Source: CAD feature listing. Evaluate the final solid. Frame: model axes, mm. Face numbers are marked on the shaded views. Round coordinates to 2 decimals unless told otherwise and drop trailing zeros. Order: outer loops, then holes, each group sorted by start corner. A loop starts at its lowest first (then second) coordinate and runs counter-clockwise, first axis right, second up. Notation, with made-up numbers: M -19,9 L 21,9 A27 cw 21,44 Z; hole C -10.75,-2.5 d10. An arc over 180 degrees is marked long. Use one line per item in the form item = value. Start each with the question number.
Q1. Section B-B (y = 0). Return the cut outline in (x, z).
Q2. Pull-direction query (Z, two-part tool) for the marked faces 1, 2 and 3; classes: pulls with the +Z half, pulls with the -Z half, needs draft (parallel to the pull), parting line crosses it, or undercut.
Q3. Contact query for flat-ended pins moving along their axis: pin 1 (3 mm diameter, centred on x = -41.5, y = -52, fed in from -Z); pin 2 (5 mm diameter, centred on y = -3.5, z = 354.5, fed in from +X); pin 3 (12 mm diameter, centred on x = 9.5, z = 331, fed in from -Y). Output: stop coordinate, or through.
Q4. Section A-A (x = 33). Return the cut outline in (y, z).
Q5. Section C-C (y = -29.5). Return the cut outline in (x, z), plus the area to 3 significant figures.
Q6. Material intervals for probe 1 along Z at (x, y) = (-42, 3.5); probe 2 along X at (y, z) = (2, 22); probe 3 along X at (y, z) = (-0.5, 442), sorted ascending.
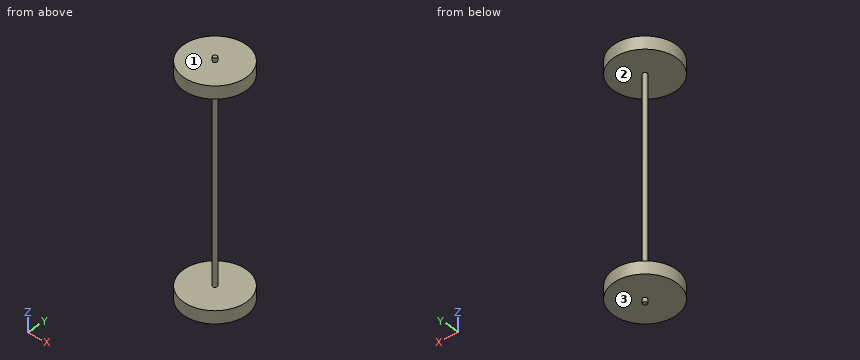
Autodesk Inventor part; units mm, degrees
ref_plane "YZ Plane" through (0, 0, 0) normal (1, 0, 0) x (0, 1, 0)
ref_plane "XZ Plane" through (0, 0, 0) normal (0, 1, 0) x (-1, 0, 0)
ref_plane "XY Plane" through (0, 0, 0) normal (0, 0, 1) x (1, 0, 0)
sketch "Skizze1" plane through (0, 0, 0) normal (0, 0, 1) x (1, 0, 0)
  line L0 (-105, 0) -> (105, 0)
  line L1 (0, -105) -> (0, 105)
  circle A0 centre (0, 0) radius 75
  dimension "d0" = 150
extrude "Extrusion1" add sketch "Skizze1" along normal blind 30
sketch "Skizze2" plane through (0, 0, 30) normal (0, 0, 1) x (1, 0, 0)
  circle A0 centre (0, 0) radius 5
  dimension "d3" = 10
extrude "Extrusion2" add sketch "Skizze2" along normal blind 480
sketch "Skizze3" plane through (0, 0, 510) normal (0, 0, 1) x (1, 0, 0)
  circle A0 centre (0, 0) radius 5
  circle A1 centre (0, 0) radius 75
extrude "Extrusion3" add sketch "Skizze3" along normal blind 30
sketch "Skizze4" plane through (0, 0, 0) normal (0, 0, -1) x (-1, 0, 0)
  circle A0 centre (0, 0) radius 5
  circle A1 centre (0, 0) radius 5
  dimension "d8" = 10
extrude "Extrusion4" add sketch "Skizze4" along normal blind 10
sketch "Skizze5" plane through (0, 0, 510) normal (0, 0, 1) x (1, 0, 0)
  circle A0 centre (0, 0) radius 5
  dimension "d11" = 10
extrude "Extrusion5" add sketch "Skizze5" along normal blind 40
properties part number "Reifen"
Results list:
q1.outline = M -75,0 L -5,0 L -5,-10 L 5,-10 L 5,0 L 75,0 L 75,30 L 5,30 L 5,510 L 75,510 L 75,540 L 5,540 L 5,550 L -5,550 L -5,540 L -75,540 L -75,510 L -5,510 L -5,30 L -75,30 Z
q2.face_1 = pulls with the +Z half
q2.face_2 = undercut
q2.face_3 = pulls with the -Z half
q3.pin_1 = 0
q3.pin_2 = 4.9
q3.pin_3 = -3.57
q4.outline = M -67.35,0 L 67.35,0 L 67.35,30 L -67.35,30 Z; M -67.35,510 L 67.35,510 L 67.35,540 L -67.35,540 Z
q5.outline = M -68.95,0 L 68.95,0 L 68.95,30 L -68.95,30 Z; M -68.95,510 L 68.95,510 L 68.95,540 L -68.95,540 Z
q5.area = 8,270 mm2
q6.probe_1 = 0 to 30, 510 to 540
q6.probe_2 = -74.97 to 74.97
q6.probe_3 = -4.97 to 4.97
